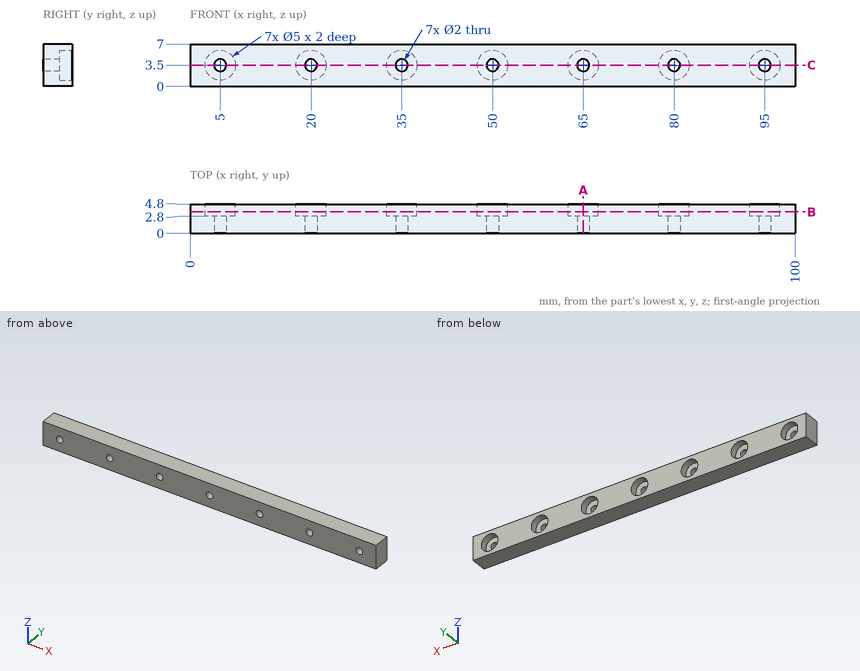
Design review of the part shown in the three views and the two pictorial views. Dimensions are in mm from the part's minimum x, y and z. Round coordinates to 2 decimals unless told otherwise and drop trailing zeros. Loops run counter-clockwise (first coordinate to the right, second up) from the corner with the lowest first, then second, coordinate; pieces in that order, holes last. Notation, with made-up numbers: M 32.25,13.25 L 91.25,13.25 A28 cw 91.25,41.25 Z; hole C 6,-22.5 d4. An arc over 180 degrees is marked long. Answer as a JSON object with one key per item and string values.
Item 1: We need section C-C on z = 3.5. State how many separate pieces and enclosed holes the cut face has, and give its area (3 significant figures).
Answer sheet:
{"separate pieces": "8", "enclosed holes": "0", "area": "371 mm^2"}
Item 2: We need section A-A on x = 65. Give the boundary of the cut face in (y, z), and give its area (3 significant figures).
Answer sheet:
{"outline": "M 0,0 L 4.8,0 L 4.8,1 L 2.8,1 L 2.8,2.5 L 0,2.5 Z; M 0,4.5 L 2.8,4.5 L 2.8,6 L 4.8,6 L 4.8,7 L 0,7 Z", "area": "18.0 mm^2"}
Item 3: Clearance check with flat-ended pins moving along their axes: P1, Ø4, axis at x = 36, z = 3, coming from the +Y side; P2, Ø4, axis at x = 95, z = 3.5, coming from the +Y side; P3, Ø1.8, axis at x = 35, z = 3.5, coming from the +Y side. State where each tip first meets the part, or that it passes through.
Answer sheet:
{"P1": "stops at y = 4.8", "P2": "stops at y = 2.8", "P3": "passes through"}
Item 4: We need section B-B on y = 3.55. Give the boundary of the cut face in (x, z), and give its area (3 significant figures).
Answer sheet:
{"outline": "M 0,0 L 100,0 L 100,7 L 0,7 Z; hole C 5,3.5 d5; hole C 20,3.5 d5; hole C 35,3.5 d5; hole C 50,3.5 d5; hole C 65,3.5 d5; hole C 80,3.5 d5; hole C 95,3.5 d5", "area": "563 mm^2"}
Item 5: Wall thickness on L1, parallel to Z at x = 50, y = 1.95; L2, parallel to Z at x = 5, y = 3.85; L3, parallel to Y at x = 94, z = 2.5: over which ranges is each line inside the solid? List them lowest first. Write a range as from..to.
Answer sheet:
{"L1": "z = 0..2.5, 4.5..7", "L2": "z = 0..1, 6..7", "L3": "y = 0..2.8"}
